Part model, mm, in its own coordinate system. Round coordinates to 2 decimals unless told otherwise and drop trailing zeros. Loops run counter-clockwise (first coordinate to the right, second up) from the corner with the lowest first, then second, coordinate; pieces in that order, holes last.
from build123d import *

# Parameters (mm, degrees)
F0_R     = 4.7625
F1_DEPTH = 9.7028
F2_R     = 2.3622
F3_DEPTH = 9.7028
F4_R     = 4.7625
F4_R_2   = 3.175
F5_DEPTH = 8.382


with BuildPart() as f1:
    # F0 (on Top) → F1 (new body)
    with BuildSketch(Plane.XY):
        Circle(F0_R)
    extrude(amount=F1_DEPTH)

    # F2 (on face) → F3 (cut, through all)
    with BuildSketch(Plane.XY.offset(9.7028)):
        Circle(F2_R)
    extrude(amount=-F3_DEPTH, mode=Mode.SUBTRACT)

    # F4 (on face) → F5 (cut)
    with BuildSketch(Plane(origin=(0, 0, 0), x_dir=(1, 0, 0), z_dir=(0, 0, -1))):
        Circle(F4_R)
        Circle(F4_R_2, mode=Mode.SUBTRACT)
    extrude(amount=-F5_DEPTH, mode=Mode.SUBTRACT)


solid = f1.part
1) Wall check: line 1 along Y through (x, z) = (0, 5) (3 decimals); line 2 along Z through (x, y) = (-3, -2.5); line 3 along X through (y, z) = (1.25, 1). Give the ranges that are in metal, low to high.
Values:
line 1: y = -3.175 to -2.362, 2.362 to 3.175
line 2: z = 8.38 to 9.7
line 3: x = -2.92 to -2, 2 to 2.92
2) Drop flat-ended pins along their axis: pin 1 Ø1 at (y, z) = (-2.5, 2.5) entering from -X; pin 2 Ø1.5 at (x, z) = (0.5, 3.5) entering from +Y (3 decimals). Give the stop position or say it passes through.
Values:
pin 1: stops at x = -2.47
pin 2: stops at y = 3.175
3) Slice it at C-C, the plane z = 7.5. Give the cut face in (x, y) (3 decimals), then the cut area to 3 significant figures.
Values:
outline: circle Ø6.35 at (0, 0); hole circle Ø4.724 at (0, 0)
area: 14.1 mm2
4) Slice it at D-D, the plane x = -3. Give the cut face in (y, z).
Values:
outline: (-3.7, 8.38) - (-1.04, 8.38) - (-1.04, 0) - (1.04, 0) - (1.04, 8.38) - (3.7, 8.38) - (3.7, 9.7) - (-3.7, 9.7) - close
5) Slice it at A-A, the plane y = 0. Give the cut face in (x, z) (1 decimal), then the cut area to 3 significant figures.
Values:
outline: (-4.8, 8.4) - (-3.2, 8.4) - (-3.2, 0) - (-2.4, 0) - (-2.4, 9.7) - (-4.8, 9.7) - close; (2.4, 0) - (3.2, 0) - (3.2, 8.4) - (4.8, 8.4) - (4.8, 9.7) - (2.4, 9.7) - close
area: 20.0 mm2
6) Mould opens along X. For faces 1 (the face through (-3.78, -2.9, 9.03)), 2 (the face through (1.27, 1.99, 4.92)), 3 (the face through (2, -2, 9.703)) say: released by +X, released by -X, zero draft, split by the parting line, or undercut.
Values:
face 1: split by the parting line
face 2: undercut
face 3: zero draft
